Design review of the part built by this model. Coordinates are the model's own, in mm. A direction names the side the tool comes from. Coordinates: 2 decimals unless noted, no trailing zeros. Write each loop counter-clockwise with the first axis right and the second up, starting at its lowest first coordinate (ties: lowest second). Pieces come first, ordered by that corner, then holes.
Q1. Clearance check with flat-ended pins moving along their axes: pin 1 Ø1.5 at (x, y) = (13, 2) entering from -Z; pin 2 Ø10 at (x, z) = (-12, 13.5) entering from -Y; pin 3 Ø5.5 at (x, y) = (-14, -3) entering from +Z; pin 4 Ø3 at (x, y) = (8, -3.5) entering from +Z. State where each tip first meets the part, or that it passes through.
Q2. Machinability: for faces 1 (the face through (14, 0, 7)), 2 (the face through (14, 0, 10)), 3 (the face through (7.885, 0.751, 18.972)), 4 (the face through (-11.5, 0, 11)), 5 (the face through (-14, 0, 7)), which of the approach directions +Z, -Z, +X, -X, +Y, -Y give a long, thin tool a straight path to every point of the face, cutting with its end or side? Answer none if there is none.
Q3. Add section C-C, the plane x = 10. Give the boundary of the cut face in (y, z).
Q4. Add section D-D, the plane y = 1. Give the boundary of the cut face in (x, z), plus the area to 3 significant figures.
Q5. Add section A-A, the plane z = 15.5. Give the boundary of the cut face in (x, y), plus the area to 3 significant figures.
Q6. Add section B-B, the plane y = -4.25. Give the boundary of the cut face in (x, z).
Q7. To check wall thickness, follow probe 1 along Z at (x, y) = (-10, -1.75); probe 2 along Z at (x, y) = (5.5, -5.5). State the ranges of each line that lie inside material, in increasing order.
from build123d import *

# Parameters (mm, degrees)
F0_W     = 23
F0_H     = 12
F1_DEPTH = 11.5
F3_DEPTH = 5.5
F4_R     = 2.5
F5_DEPTH = 4
F6_W     = 5
F6_H     = 3
F7_DEPTH = 12


with BuildPart() as f1:
    # F0 (on Top) → F1 (new body, symmetric)
    with BuildSketch(Plane.XY):
        Rectangle(F0_W, F0_H)
    extrude(amount=F1_DEPTH, both=True)

    # F2 (on face) → F3 (join)
    with BuildSketch(Plane.XY.offset(11.5)):
        with BuildLine():
            ThreePointArc((5.5, -6), (9.7426406871, -4.2426406871), (11.5, 0))
            ThreePointArc((11.5, 0), (9.7426406871, 4.2426406871), (5.5, 6))
            ThreePointArc((5.5, 6), (2.0238066485, 4.8904069139), (-0.1666666667, 1.9720265944))
            ThreePointArc((-0.1666666667, 1.9720265944), (1.0275252317, 1.2909944487), (1.5, 0))
            ThreePointArc((1.5, 0), (1.0275252317, -1.2909944487), (-0.1666666667, -1.9720265944))
            ThreePointArc((-0.1666666667, -1.9720265944), (2.0238066485, -4.8904069139), (5.5, -6))
        make_face()
        with BuildLine():
            ThreePointArc((1.5, 0), (1.0275252317, 1.2909944487), (-0.1666666667, 1.9720265944))
            ThreePointArc((-0.1666666667, 1.9720265944), (-0.5, 0), (-0.1666666667, -1.9720265944))
            ThreePointArc((-0.1666666667, -1.9720265944), (1.0275252317, -1.2909944487), (1.5, 0))
        make_face()
        with BuildLine():
            ThreePointArc((-0.1666666667, -1.9720265944), (-0.5, 0), (-0.1666666667, 1.9720265944))
            ThreePointArc((-0.1666666667, 1.9720265944), (-2.5, 0), (-0.1666666667, -1.9720265944))
        make_face()
    extrude(amount=F3_DEPTH)

    # F4 (on face) → F5 (join)
    with BuildSketch(Plane.XY.offset(17)):
        with Locations((5.5, 0)):
            Circle(F4_R)
    extrude(amount=F5_DEPTH)

    # F6 (on face) → F7 (join)
    with BuildSketch(Plane.XZ.offset(6)):
        with Locations((-14, 8.5)):
            Rectangle(F6_W, F6_H)
        with Locations((14, 8.5)):
            Rectangle(F6_W, F6_H)
    extrude(amount=-F7_DEPTH)


solid = f1.part
Here are the results:
1. pin 1: stops at z = 7
1. pin 2: stops at y = -6
1. pin 3: stops at z = 11.5
1. pin 4: stops at z = 17
2. face 1: -Z, +X, +Y, -Y
2. face 2: +Z, +X, +Y, -Y
2. face 3: +Z
2. face 4: +Z, -X, +Y, -Y
2. face 5: -Z, -X, +Y, -Y
3. outline: (-6, -11.5) - (6, -11.5) - (6, 11.5) - (3.97, 11.5) - (3.97, 17) - (-3.97, 17) - (-3.97, 11.5) - (-6, 11.5) - close
4. outline: (-16.5, 7) - (-11.5, 7) - (-11.5, -11.5) - (11.5, -11.5) - (11.5, 7) - (16.5, 7) - (16.5, 10) - (11.5, 10) - (11.5, 11.5) - (11.42, 11.5) - (11.42, 17) - (7.79, 17) - (7.79, 21) - (3.21, 21) - (3.21, 17) - (-2.23, 17) - (-2.23, 11.5) - (-11.5, 11.5) - (-11.5, 10) - (-16.5, 10) - close
4. area: 652 mm2
5. outline: (-0.17, -1.97) arc R6 ccw (long way) to (-0.17, 1.97) arc R2 ccw (long way) to start
5. area: 120 mm2
6. outline: (-16.5, 7) - (-11.5, 7) - (-11.5, -11.5) - (11.5, -11.5) - (11.5, 7) - (16.5, 7) - (16.5, 10) - (11.5, 10) - (11.5, 11.5) - (9.74, 11.5) - (9.74, 17) - (1.26, 17) - (1.26, 11.5) - (-11.5, 11.5) - (-11.5, 10) - (-16.5, 10) - close
7. probe 1: z = -11.5 to 11.5
7. probe 2: z = -11.5 to 17
